from build123d import *

# Parameters (mm, degrees)
BOSS_EXTRUDE1_DEPTH = 1


with BuildPart() as part:
    # Sketch1 → Revolve1 (revolve)
    with BuildSketch(Plane.XY):
        Polygon((0, 0), (0, 1.35), (7.25, 1.35), (7.25, 2.65), (0, 2.65), (0, 3.15), (7.25, 3.15), (7.25, 4.45), (0, 4.45), (0, 4.95), (7.25, 4.95), (7.25, 5.85), (8.25, 5.85), (8.25, 0), align=None)
    revolve(axis=Axis((8.25, 0, 0), (-1, 0, 0)))

    # Sketch2 → Boss-Extrude1 (add)
    with BuildSketch(Plane(origin=(8.25, 0, 0), x_dir=(0, 0, -1), z_dir=(1, 0, 0))):
        Polygon((5.94, -3.429460599), (5.94, 3.429460599), (0, 6.858921198), (-5.94, 3.429460599), (-5.94, -3.429460599), (0, -6.858921198), align=None)
    extrude(amount=-BOSS_EXTRUDE1_DEPTH)

    # Mirror1: part across face


with BuildPart() as part_1:
    add(part.part)
    add(part.part.mirror(Plane(origin=(8.25, 0, 0), x_dir=(0, 0, 1), z_dir=(1, 0, 0))))


solid = part_1.part
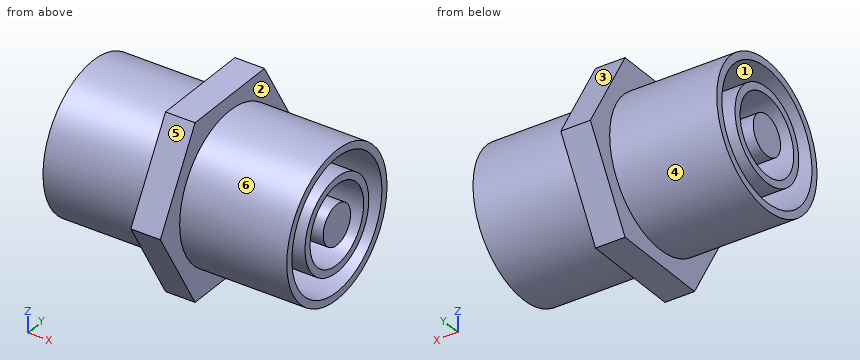
Verification items for the finished model (mm, model axes). Face numbers are marked on the shaded views. A direction names the side the tool comes from. Coordinates: 2 decimals unless noted, no trailing zeros. Order: outer loops, then holes, each group sorted by start corner. A loop starts at its lowest first (then second) coordinate and runs counter-clockwise, first axis right, second up. Notation, with made-up numbers: M 88.25,67.25 L 133.25,67.25 A33 cw 133.25,99.25 Z; hole C 82,77.25 d1. An arc over 180 degrees is marked long. One line per item, written item: value. Start each with the question number.
Item 1: Sectioned sample at A-A (x = 12). Enter the section's corners in (y, z).
Item 2: Scan lines: probe 1 along Y at (x, z) = (12.25, 0); probe 2 along Y at (x, z) = (12, -2.25). Record each from-to range of solid material in increasing order.
Item 3: Sectioned sample at B-B (z = -3.5). Enter the section's corners in (x, y).
Item 4: Gauge pin test, flat ends, axial feed: pin 1 (1.5 mm diameter, centred on x = 2.5, z = 2, fed in from -Y); pin 2 (3 mm diameter, centred on x = 12.5, y = 1.5, fed in from +Z); pin 3 (3 mm diameter, centred on x = 12.5, y = 0, fed in from -Z). Record the tip position at first contact, or that the pin passes through.
Item 5: Mould release check, pull along Y, two halves, no side actions. Record for the marked faces 1, 2 and 3: released by +Y, released by -Y, zero draft, split by the parting line, or undercut.
Item 6: Access from +Z, -Z, +X, -X, +Y, -Y to the whole of each face (thin tool, end or side, straight path). Record for the marked faces 4, 5 and 6.
Conclusion:
1. outline: C 0,0 d9.9; C 0,0 d6.3; C 0,0 d2.7; hole C 0,0 d8.9; hole C 0,0 d5.3
2. probe 1: y = -4.95 to -4.45, -3.15 to -2.65, -1.35 to 1.35, 2.65 to 3.15, 4.45 to 4.95
2. probe 2: y = -4.41 to -3.84, -2.2 to -1.4, 1.4 to 2.2, 3.84 to 4.41
3. outline: M 0,-3.5 L 7.25,-3.5 L 7.25,-4.84 L 9.25,-4.84 L 9.25,-3.5 L 16.5,-3.5 L 16.5,-2.75 L 9.25,-2.75 L 9.25,2.75 L 16.5,2.75 L 16.5,3.5 L 9.25,3.5 L 9.25,4.84 L 7.25,4.84 L 7.25,3.5 L 0,3.5 L 0,2.75 L 7.25,2.75 L 7.25,-2.75 L 0,-2.75 Z
4. pin 1: stops at y = -4.79
4. pin 2: stops at z = 4.95
4. pin 3: stops at z = -4.95
5. face 1: undercut
5. face 2: zero draft
5. face 3: released by +Y
6. face 4: -X
6. face 5: +Z, +X, -X, -Y
6. face 6: +X
